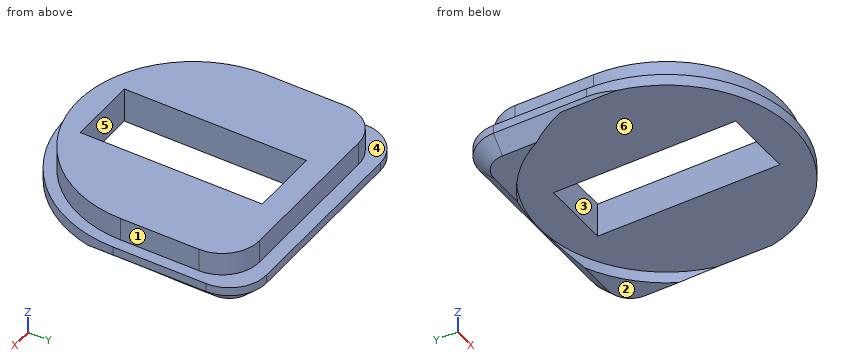
```python
from build123d import *

# Parameters (mm, degrees)
F1_DEPTH    = 3.175
F3_DEPTH    = 3.175
F5_DEPTH    = 1.5875
F6_W        = 9.6138492227
F6_H        = 25.0137764961
F7_DEPTH    = 25.4
F8_R        = 5.08
F9_T1_DEPTH = 21.5230971591
F9_T3_DEPTH = 24.765
F9_T6_ANGLE = 90
F9_T8_ANGLE = 90


# Not quite as in the source:
# - a fillet or chamfer that OpenCascade refuses, or shapes differently, is made with other operations: its cross-section is extruded or revolved along the edge and cut away or added


with BuildPart() as f1:
    # F0 (on Top) → F1 (new body)
    with BuildSketch(Plane.XY):
        with BuildLine():
            ThreePointArc((-17.4625, 0), (0, -17.4625), (17.4625, 0))
            ThreePointArc((17.4625, 0), (0, 17.4625), (-17.4625, 0))
        make_face()
        with BuildLine():
            ThreePointArc((-17.4625, 0), (0, 17.4625), (17.4625, 0))
            Line((17.4625, 0), (17.4625, 17.859375))
            Line((17.4625, 17.859375), (-17.4625, 17.859375))
            Line((-17.4625, 17.859375), (-17.4625, 0))
        make_face()
    extrude(amount=F1_DEPTH)

    # F2 (on face) → F3 (join)
    with BuildSketch(Plane.XY.offset(3.175)):
        with BuildLine():
            ThreePointArc((-5.44e-08, 15.875), (-11.2253201706, 11.2253201321), (-15.875, 0))
            ThreePointArc((-15.875, 0), (0, -15.875), (15.875, 0))
            ThreePointArc((15.875, 0), (11.2253201321, 11.2253201706), (-5.44e-08, 15.875))
        make_face()
        with BuildLine():
            Line((-15.875, 15.875), (-15.875, 0))
            ThreePointArc((-15.875, 0), (-11.2253201706, 11.2253201321), (-5.44e-08, 15.875))
            Line((-5.44e-08, 15.875), (-15.875, 15.875))
        make_face()
        with BuildLine():
            ThreePointArc((-5.44e-08, 15.875), (11.2253201321, 11.2253201706), (15.875, 0))
            Line((15.875, 0), (15.875, 15.875))
            Line((15.875, 15.875), (-5.44e-08, 15.875))
        make_face()
    extrude(amount=F3_DEPTH)

    # F4 (on face) → F5 (cut)
    with BuildSketch(Plane(origin=(0, 0, 0), x_dir=(1, 0, 0), z_dir=(0, 0, -1))):
        with BuildLine():
            ThreePointArc((-17.4625, 0), (0, -17.4625), (17.4625, 0))
            ThreePointArc((17.4625, 0), (0, 17.4625), (-17.4625, 0))
        make_face()
    extrude(amount=-F5_DEPTH, mode=Mode.SUBTRACT)

    # F6 (on face) → F7 (cut)
    with BuildSketch(Plane(origin=(0, 0, 1.5875), x_dir=(1, 0, 0), z_dir=(0, 0, -1))):
        Rectangle(F6_W, F6_H)
    extrude(amount=-F7_DEPTH, mode=Mode.SUBTRACT)

    # F8
    f8_edges = [f1.edges().sort_by_distance(p)[0] for p in [
        (17.4625, 17.859375, 1.5875),
        (-17.4625, 17.859375, 1.5875),
        (-15.875, 15.875, 4.7625),
        (15.875, 15.875, 4.7625),
    ]]
    fillet(f8_edges, radius=F8_R)

    # F9: chamfer of 2 on 2 edges, made by hand

    # F9_s2 → F9_t1 (cut)
    with BuildSketch(Plane.XZ.offset(-12.779375)):
        Polygon((17.4625, 2), (15.4625, 0), (17.4625, 0), align=None)
        Polygon((-15.4625, 0), (-17.4625, 2), (-17.4625, 0), align=None)
    extrude(amount=F9_T1_DEPTH, mode=Mode.SUBTRACT)

    # F9_s4 → F9_t3 (cut)
    with BuildSketch(Plane.YZ.offset(-12.3825)):
        Polygon((15.859375, 0), (17.859375, 2), (17.859375, 0), align=None)
    extrude(amount=F9_T3_DEPTH, mode=Mode.SUBTRACT)

    # F9_s5 → F9_t6 (revolve, cut)
    with BuildSketch(Plane.XZ.offset(-12.779375)):
        Polygon((15.4625, 0), (17.4625, 2), (17.4625, 0), align=None)
    revolve(axis=Axis((12.3825, 12.779375, 0), (0, 0, 1)), revolution_arc=F9_T6_ANGLE, mode=Mode.SUBTRACT)

    # F9_s7 → F9_t8 (revolve, cut)
    with BuildSketch(Plane.YZ.offset(-12.3825)):
        Polygon((15.859375, 0), (17.859375, 2), (17.859375, 0), align=None)
    revolve(axis=Axis((-12.3825, 12.779375, 0), (0, 0, 1)), revolution_arc=F9_T8_ANGLE, mode=Mode.SUBTRACT)


solid = f1.part
```
Source: CAD feature listing. Evaluate the final solid. Frame: model axes, mm. Face numbers are marked on the shaded views. A direction names the side the tool comes from. Round coordinates to 2 decimals unless told otherwise and drop trailing zeros. Loops run counter-clockwise (first coordinate to the right, second up) from the corner with the lowest first, then second, coordinate; pieces in that order, holes last.
1. Section query C-C on z = 5.5. Output: boundary loops of the cut face in (x, y) (3 decimals), and give its area (3 significant figures).
2. Mould query, pull axis X, two halves, no side actions, for the marked faces 1, 2 and 3. Classes: released by +X, released by -X, zero draft, split by the parting line, or undercut.
3. Ray query, L1, parallel to X at y = 10, z = 5.25 (3 decimals); L2, parallel to Z at x = 9, y = -13; L3, parallel to X at y = -6, z = 3. Return the intervals inside material, ascending.
4. Contact query for flat-ended pins moving along their axis: pin 1 (2 mm diameter, centred on x = 14, y = -11, fed in from -Z); pin 2 (2.5 mm diameter, centred on x = 3, z = 4.5, fed in from +Y) (3 decimals); pin 3 (1.5 mm diameter, centred on y = -13, z = 1, fed in from +X). Output: stop coordinate, or through.
5. Access query for the marked faces 4, 5 and 6. Directions: +Z, -Z, +X, -X, +Y, -Y. A direction counts if a zero-diameter tool reaches every point of the face in a straight line with its end or side. Return the directions, or none.
Answers below:
1. outline: (-15.875, 0) arc R15.875 ccw to (15.875, 0) - (15.875, 10.795) arc R5.08 ccw to (10.795, 15.875) - (-10.795, 15.875) arc R5.08 ccw to (-15.875, 10.795) - close; hole (-4.807, -12.507) - (4.807, -12.507) - (4.807, 12.507) - (-4.807, 12.507) - close
1. area: 648 mm2
2. face 1: released by +X
2. face 2: zero draft
2. face 3: undercut
3. L1: x = -15.875 to -4.807, 4.807 to 15.875
3. L2: z = 1.59 to 6.35
3. L3: x = -16.4 to -4.81, 4.81 to 16.4
4. pin 1: stops at z = 1.59
4. pin 2: stops at y = 15.875
4. pin 3: stops at x = 12.16
5. face 4: +Z
5. face 5: +Z, -Z
5. face 6: -Z, -Y
